Design review of the part built by this model. Coordinates are the model's own, in mm. Face numbers are marked on the shaded views. A direction names the side the tool comes from. Coordinates: 2 decimals unless noted, no trailing zeros. Loops run counter-clockwise (first coordinate to the right, second up) from the corner with the lowest first, then second, coordinate; pieces in that order, holes last.
Q1. Add section C-C on x = 129.5. Give the boundary of the cut face in (y, z).
Q2. Add section D-D on z = 14.5. Give the boundary of the cut face in (x, y).
Q3. For P1, Ø3, axis at x = 2, z = -18.5, coming from the -Y side; P2, Ø3, axis at y = -111, z = -21, coming from the -X side; P3, Ø6, axis at x = 113.5, z = 38, coming from the -Y side, all flat-tipped, find the tip position at first contact; note any pin that passes through.
Q4. Draft analysis for pull direction Y (two halves, no side actions). For the marked faces 1, 2 and 3, state which applies: released by +Y, released by -Y, zero draft, split by the parting line, or undercut.
Q5. Machinability: for the marked faces 4, 5 and 6, which of the approach directions +Z, -Z, +X, -X, +Y, -Y give a long, thin tool a straight path to every point of the face, cutting with its end or side? Answer none if there is none.
Q6. Wall thickness on probe 1 along X at (y, z) = (-46, 33); probe 2 along Y at (x, z) = (-7.5, -10); probe 3 along X at (y, z) = (-87, -2.5): over which ranges is each line inside the solid? List them lowest first.
Q7. Add section A-A on z = 46.5. Give the number of separate pieces and of enclosed holes in the cut face, and give its area (3 significant figures).
```python
from build123d import *
from build123d.topology import SkipClean

# Parameters (mm, degrees)
SKETCH1_R           = 150
BOSS_EXTRUDE1_DEPTH = 30
SKETCH2_R           = 135
SKETCH2_R_2         = 120
SKETCH2_R_3         = 105
SKETCH2_R_4         = 90
SKETCH2_R_5         = 75
SKETCH2_R_6         = 60
SKETCH2_R_7         = 45
SKETCH2_R_8         = 30
SKETCH2_R_9         = 15
BOSS_EXTRUDE2_DEPTH = 30
BOSS_EXTRUDE3_START = 30
SKETCH3_R           = 135
SKETCH3_R_2         = 115
SKETCH3_R_3         = 75
SKETCH3_R_4         = 55
SKETCH3_R_5         = 35
SKETCH3_R_6         = 15
BOSS_EXTRUDE3_DEPTH = 30
BOSS_EXTRUDE4_START = 30
BOSS_EXTRUDE4_DEPTH = 30


with BuildPart() as part:
    # Sketch1 → Boss-Extrude1 (new body)
    with BuildSketch(Plane.XY):
        Circle(SKETCH1_R)
    extrude(amount=BOSS_EXTRUDE1_DEPTH)

    # Sketch2 → Boss-Extrude2 (add)
    # profile 1 of 5: a face of its own
    with BuildSketch(Plane.XY.offset(30)):
        Circle(SKETCH2_R)
        Circle(SKETCH2_R_2, mode=Mode.SUBTRACT)
    # profile 2 of 5: a face of its own
    with BuildSketch(Plane.XY.offset(30)):
        Circle(SKETCH2_R_3)
        Circle(SKETCH2_R_4, mode=Mode.SUBTRACT)
    # profile 3 of 5: a face of its own
    with BuildSketch(Plane.XY.offset(30)):
        Circle(SKETCH2_R_5)
        Circle(SKETCH2_R_6, mode=Mode.SUBTRACT)
    # profile 4 of 5: a face of its own
    with BuildSketch(Plane.XY.offset(30)):
        Circle(SKETCH2_R_7)
        Circle(SKETCH2_R_8, mode=Mode.SUBTRACT)
    # profile 5 of 5: a face of its own
    with BuildSketch(Plane.XY.offset(30)):
        Circle(SKETCH2_R_9)
    extrude(amount=BOSS_EXTRUDE2_DEPTH)

    # Sketch3 → Boss-Extrude3 (add)
    # profile 1 of 3: a face of its own
    with BuildSketch(Plane(origin=(0, 0, 0), x_dir=(-1, 0, 0), z_dir=(0, 0, -1)).offset(BOSS_EXTRUDE3_START)):
        with Locations(Location((0, 0, 0), (0, 0, 180))):
            Circle(SKETCH3_R)
        Circle(SKETCH3_R_2, mode=Mode.SUBTRACT)
    # profile 2 of 3: a face of its own
    with BuildSketch(Plane(origin=(0, 0, 0), x_dir=(-1, 0, 0), z_dir=(0, 0, -1)).offset(BOSS_EXTRUDE3_START)):
        with Locations(Location((0, 0, 0), (0, 0, 180))):
            Circle(SKETCH3_R_3)
        Circle(SKETCH3_R_4, mode=Mode.SUBTRACT)
    # profile 3 of 3: a face of its own
    with BuildSketch(Plane(origin=(0, 0, 0), x_dir=(-1, 0, 0), z_dir=(0, 0, -1)).offset(BOSS_EXTRUDE3_START)):
        with Locations(Location((0, 0, 0), (0, 0, 180))):
            Circle(SKETCH3_R_5)
        with Locations(Location((0, 0, 0), (0, 0, 180))):
            Circle(SKETCH3_R_6, mode=Mode.SUBTRACT)
    extrude(amount=-BOSS_EXTRUDE3_DEPTH)

    # Sketch4 → Boss-Extrude4 (add)
    with SkipClean():  # the faces are left unmerged after this step: merging them gives an invalid solid
        with BuildSketch(Plane(origin=(0, 0, 0), x_dir=(-1, 0, 0), z_dir=(0, 0, -1)).offset(BOSS_EXTRUDE4_START)):
            with BuildLine():
                Line((-5.347315923, 50), (5.347315923, 50))
                Line((5.347315923, 50), (17.5, 148.975669154))
                ThreePointArc((17.5, 148.975669154), (0, 150), (-17.5, 148.975669154))
                Line((-17.5, 148.975669154), (-5.347315923, 50))
            make_face()
            with BuildLine():
                Line((50, 5.347315923), (148.975669154, 17.5))
                ThreePointArc((148.975669154, 17.5), (150, 0), (148.975669154, -17.5))
                Line((148.975669154, -17.5), (50, -5.347315923))
                Line((50, -5.347315923), (50, 5.347315923))
            make_face()
            with BuildLine():
                Line((5.347315923, -50), (17.5, -148.975669154))
                ThreePointArc((17.5, -148.975669154), (0, -150), (-17.5, -148.975669154))
                Line((-17.5, -148.975669154), (-5.347315923, -50))
                Line((-5.347315923, -50), (5.347315923, -50))
            make_face()
            with BuildLine():
                Line((-50, -5.347315923), (-148.975669154, -17.5))
                ThreePointArc((-148.975669154, -17.5), (-150, 0), (-148.975669154, 17.5))
                Line((-148.975669154, 17.5), (-50, 5.347315923))
                Line((-50, 5.347315923), (-50, -5.347315923))
            make_face()
        extrude(amount=-BOSS_EXTRUDE4_DEPTH)


solid = part.part
```
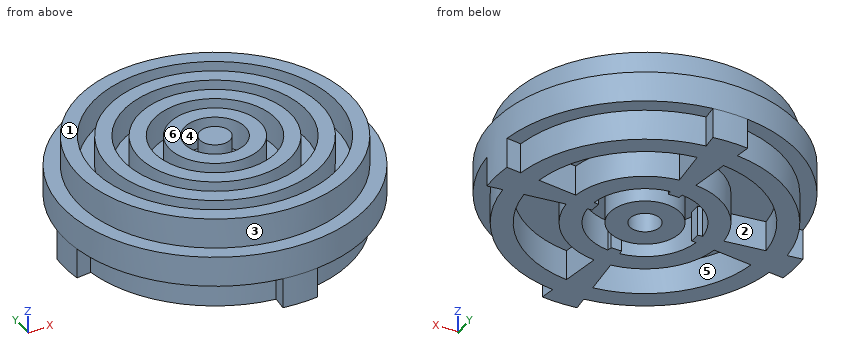
Entries:
1. outline: (-75.7, 0) - (-38.14, 0) - (-38.14, -30) - (38.14, -30) - (38.14, 0) - (75.7, 0) - (75.7, 30) - (38.14, 30) - (38.14, 60) - (-38.14, 60) - (-38.14, 30) - (-75.7, 30) - close
2. outline: circle Ø300 at (0, 0)
3. P1: stops at y = -150
3. P2: stops at x = -78.96
3. P3: stops at y = -77.55
4. face 1: zero draft
4. face 2: undercut
4. face 3: split by the parting line
5. face 4: +Z
5. face 5: -Z
5. face 6: +Z, +X, -X, +Y, -Y
6. probe 1: x = -126.92 to -110.83, -94.39 to -77.36, -59.24 to -38.52, 38.52 to 59.24, 77.36 to 94.39, 110.83 to 126.92
6. probe 2: y = -149.81 to -54.49, -34.19 to -12.99, 12.99 to 34.19, 54.49 to 149.81
6. probe 3: x = -103.23 to -75.21, -9.89 to 9.89, 75.21 to 103.23
7. separate pieces: 5
7. enclosed holes: 4
7. area: 31,800 mm2
